Model file for the job. Use its own axes, mm. A direction names the side the tool comes from. Coordinates: 2 decimals unless noted, no trailing zeros. Write each loop counter-clockwise with the first axis right and the second up, starting at its lowest first coordinate (ties: lowest second). Pieces come first, ordered by that corner, then holes. Notation, with made-up numbers: (43.5, 24.5) - (53.5, 24.5) arc R10 ccw to (53.5, 36.5) - close; hole circle Ø4 at (1.5, 8). An arc over 180 degrees is marked (long way). Put each result on its own line as item: value. Start each with the question number.
1. Which spindle directions (+Z, -Z, +X, -X, +Y, -Y) get a long thin tool onto all of the face, cutting with end or side? Do faces 1 (the face through (0.64, 7.574, 28.444)), 2 (the face through (0, 6, 32.5)), 3 (the face through (2, 4, 22.5)), 4 (the face through (-6, 0, -32.6)). Say none if no direction does.
2. Saw through at D-D, the plane y = -10.5. Write the cut outline in (x, z).
3. Drill centre lines: L1, parallel to Z at x = 4.5, y = -14.5; L2, parallel to Z at x = 7, y = 3; L3, parallel to Y at x = -0.5, z = -9. Where is each one in solid material? Low to high. Write a range as from..to.
4. Saw through at A-A, the plane y = 0. Write the cut outline in (x, z), plus the area to 3 significant figures.
5. Drop flat-ended pins along their axis: P1, Ø3, axis at x = 12.5, y = -3.5, coming from the -Z side; P2, Ø4, axis at x = 7.5, z = -22, coming from the -Y side; P3, Ø1, axis at y = -9.5, z = 4, coming from the -X side. Give the stop position or say it passes through.
6. Saw through at C-C, the plane z = 8.5. Write the cut outline in (x, y).
7. Pull direction Z, two halves, no side cores. Call faces 5 (the face through (0.91, -0.7, -36.43)), 6 (the face through (0, 0, 20)), 7 (the face through (0, 0, -38.1)): released by +Z, released by -Z, zero draft, split by the parting line, or undercut.
8. Saw through at B-B, the plane x = 0. Write the cut outline in (y, z).
```python
from build123d import *

# Parameters (mm, degrees)
SKETCH1_R           = 16.5
BOSS_EXTRUDE1_DEPTH = 20
SKETCH2_R           = 13.85
BOSS_EXTRUDE2_DEPTH = 32.6
SKETCH3_R           = 5
BOSS_EXTRUDE3_DEPTH = 2.2
SKETCH4_R           = 1.15
BOSS_EXTRUDE4_DEPTH = 3.3
SKETCH5_R           = 5
BOSS_EXTRUDE5_DEPTH = 2.5
SKETCH6_R           = 2.5
BOSS_EXTRUDE6_DEPTH = 10
CUT_EXTRUDE1_START  = -8
CUT_EXTRUDE1_DEPTH  = 8


with BuildPart() as part:
    # Sketch1 → Boss-Extrude1 (new body)
    with BuildSketch(Plane.XY):
        Circle(SKETCH1_R)
    extrude(amount=BOSS_EXTRUDE1_DEPTH)

    # Sketch2 → Boss-Extrude2 (add)
    with BuildSketch(Plane(origin=(0, 0, 0), x_dir=(-1, 0, 0), z_dir=(0, 0, -1))):
        Circle(SKETCH2_R)
    extrude(amount=BOSS_EXTRUDE2_DEPTH)

    # Sketch3 → Boss-Extrude3 (add)
    with BuildSketch(Plane(origin=(0, 0, -32.6), x_dir=(-1, 0, 0), z_dir=(0, 0, -1))):
        Circle(SKETCH3_R)
    extrude(amount=BOSS_EXTRUDE3_DEPTH)

    # Sketch4 → Boss-Extrude4 (add)
    with BuildSketch(Plane(origin=(0, 0, -34.8), x_dir=(-1, 0, 0), z_dir=(0, 0, -1))):
        Circle(SKETCH4_R)
    extrude(amount=BOSS_EXTRUDE4_DEPTH)

    # Sketch5 → Boss-Extrude5 (add)
    with BuildSketch(Plane.XY.offset(20)):
        with Locations((0, 6)):
            Circle(SKETCH5_R)
    extrude(amount=BOSS_EXTRUDE5_DEPTH)

    # Sketch6 → Boss-Extrude6 (add)
    with BuildSketch(Plane.XY.offset(22.5)):
        with Locations((0, 6)):
            Circle(SKETCH6_R)
    extrude(amount=BOSS_EXTRUDE6_DEPTH)

    # Sketch7 → Cut-Extrude1 (cut)
    with BuildSketch(Plane.XY.offset(32.5).offset(CUT_EXTRUDE1_START)):
        with BuildLine():
            Line((-1.024171461, 8.280586069), (2.352192857, 6.84686998))
            ThreePointArc((2.352192857, 6.84686998), (0.977136461, 8.301131099), (-1.024171461, 8.280586069))
        make_face()
    extrude(amount=CUT_EXTRUDE1_DEPTH, mode=Mode.SUBTRACT)


solid = part.part
```
Final values:
1. face 1: +Z, +X, +Y
1. face 2: +Z, +X, -X, +Y, -Y
1. face 3: +Z
1. face 4: -Z
2. outline: (-12.73, 0) - (-9.03, 0) - (-9.03, -32.6) - (9.03, -32.6) - (9.03, 0) - (12.73, 0) - (12.73, 20) - (-12.73, 20) - close
3. L1: z = 0..20
3. L2: z = -32.6..20
3. L3: y = -13.84..13.84
4. outline: (-16.5, 0) - (-13.85, 0) - (-13.85, -32.6) - (-5, -32.6) - (-5, -34.8) - (-1.15, -34.8) - (-1.15, -38.1) - (1.15, -38.1) - (1.15, -34.8) - (5, -34.8) - (5, -32.6) - (13.85, -32.6) - (13.85, 0) - (16.5, 0) - (16.5, 20) - (-16.5, 20) - close
4. area: 1,590 mm²
5. P1: stops at z = -32.6
5. P2: stops at y = -12.71
5. P3: stops at x = -13.83
6. outline: circle Ø33 at (0, 0)
7. face 5: zero draft
7. face 6: released by +Z
7. face 7: released by -Z
8. outline: (-16.5, 0) - (-13.85, 0) - (-13.85, -32.6) - (-5, -32.6) - (-5, -34.8) - (-1.15, -34.8) - (-1.15, -38.1) - (1.15, -38.1) - (1.15, -34.8) - (5, -34.8) - (5, -32.6) - (13.85, -32.6) - (13.85, 0) - (16.5, 0) - (16.5, 20) - (11, 20) - (11, 22.5) - (8.5, 22.5) - (8.5, 24.5) - (7.85, 24.5) - (7.85, 32.5) - (3.5, 32.5) - (3.5, 22.5) - (1, 22.5) - (1, 20) - (-16.5, 20) - close
